Part print with two shaded views. Sizes in mm from the minimum x, y, z corner. Coordinates: 2 decimals unless noted, no trailing zeros. Loops run counter-clockwise (first coordinate to the right, second up) from the corner with the lowest first, then second, coordinate; pieces in that order, holes last.
Item 1: Mould opens along X. For the marked faces 1, 2, 3 and 4 say: released by +X, released by -X, zero draft, split by the parting line, or undercut.
Item 2: Drill centre lines: line 1 along X through (y, z) = (2.1, 12.5); line 2 along X through (y, z) = (3.8, 9.5); line 3 along Y through (x, z) = (10.25, 17.25). Where is each one in solid material? Low to high.
Item 3: Cut at C-C (y = 3.45). List the corners of the cut face in (x, z).
Item 4: Cut at A-A (x = 12.5). List the corners of the cut face in (y, z), and give its area (3 significant figures).
Item 5: Cut at B-B (z = 12.5). List the corners of the cut face in (x, y), and give its area (3 significant figures).
Item 6: Cut at D-D (y = 0.5). List the corners of the cut face in (x, z), and give its area (3 significant figures).
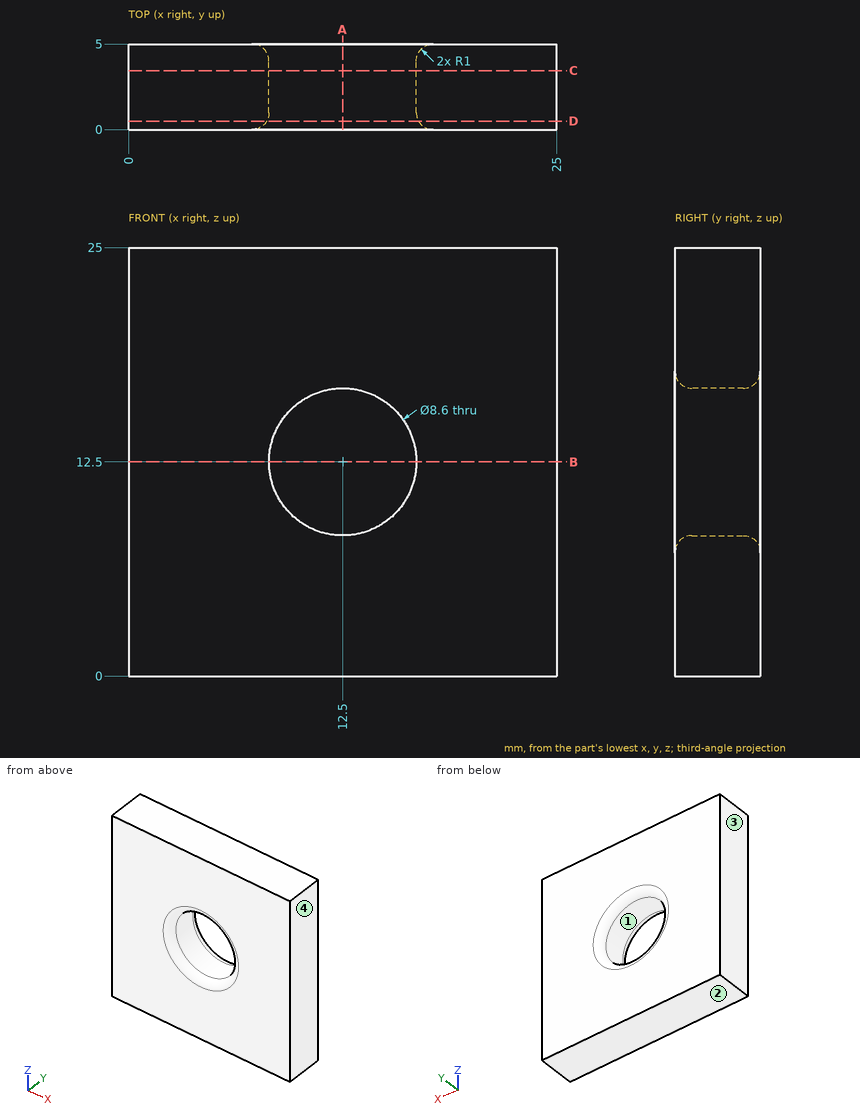
Filled sheet:
1. face 1: undercut
1. face 2: zero draft
1. face 3: released by -X
1. face 4: released by +X
2. line 1: x = 0 to 8.2, 16.8 to 25
2. line 2: x = 0 to 9.42, 15.58 to 25
2. line 3: y = 0 to 5
3. outline: (0, 0) - (25, 0) - (25, 25) - (0, 25) - close; hole circle Ø8.6 at (12.5, 12.5)
4. outline: (0, 0) - (5, 0) - (5, 7.2) arc R1 ccw to (4, 8.2) - (1, 8.2) arc R1 ccw to (0, 7.2) - close; (0, 17.8) arc R1 ccw to (1, 16.8) - (4, 16.8) arc R1 ccw to (5, 17.8) - (5, 25) - (0, 25) - close
4. area: 81.1 mm2
5. outline: (0, 0) - (7.2, 0) arc R1 ccw to (8.2, 1) - (8.2, 4) arc R1 ccw to (7.2, 5) - (0, 5) - close; (16.8, 1) arc R1 ccw to (17.8, 0) - (25, 0) - (25, 5) - (17.8, 5) arc R1 ccw to (16.8, 4) - close
5. area: 81.1 mm2
6. outline: (0, 0) - (25, 0) - (25, 25) - (0, 25) - close; hole circle Ø8.87 at (12.5, 12.5)
6. area: 563 mm2
